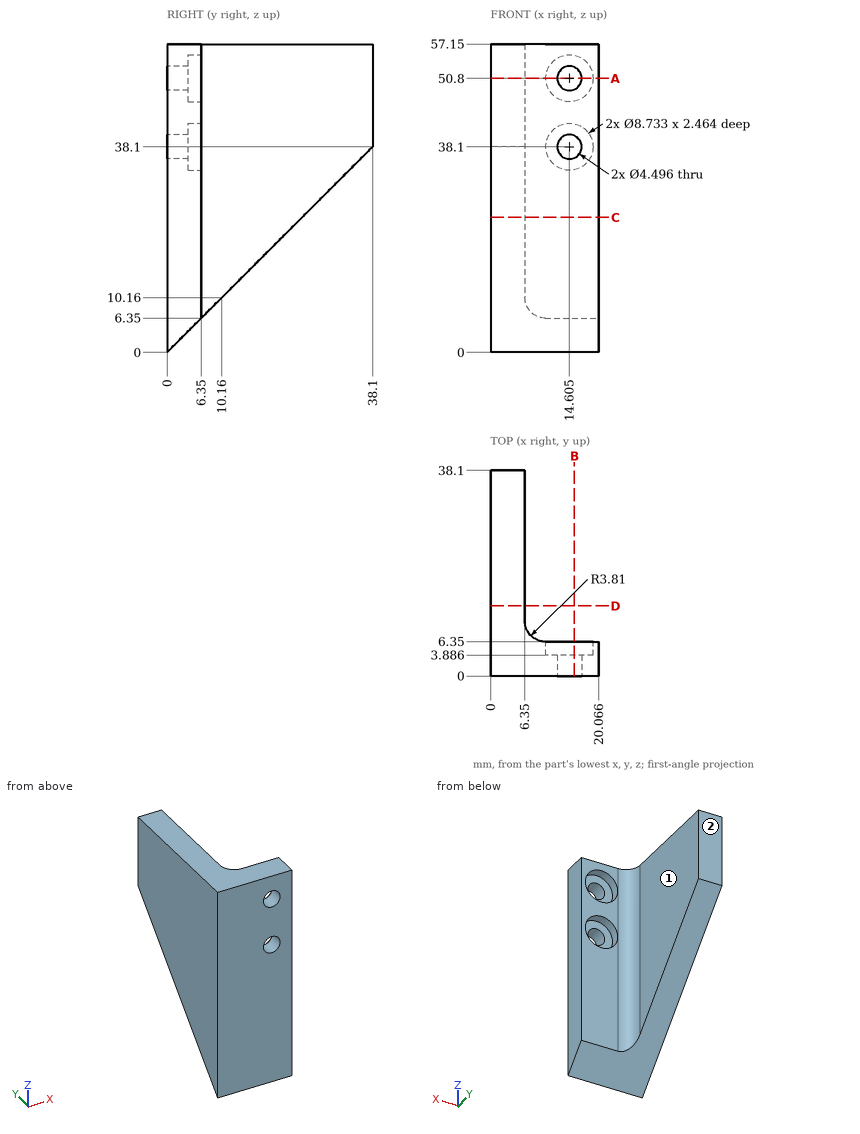
Could you check a few things on this drawing? It's one solid part, dimensions in mm from its lowest x, y, z. A direction names the side the tool comes from. Give positions to 0.01 mm unless a question says otherwise; leave off trailing zeros. Write each loop counter-clockwise with the first axis right and the second up, starting at its lowest first coordinate (ties: lowest second). Pieces come first, ordered by that corner, then holes. Notation, with made-up numbers: (76.5, 10.5) - (85.5, 10.5) arc R26 cw to (85.5, 46.5) - close; hole circle Ø10 at (33, 21). An arc over 180 degrees is marked (long way). Use CSV: the item, a comma, the result in double quotes. Start each with the question number.
Item 1: If I drill on line 1 along X through (y, z) = (5, 38); line 2 along X through (y, z) = (2.1, 38.1); line 3 along Y through (x, z) = (17.25, 32.5), over which ranges is the centre line in solid material (lowest first)?
Item 2: I want a section at D-D, the plane y = 13. Please give me the cut outline in (x, z), then the cut area to 3 significant figures.
Item 3: I want a section at A-A, the plane z = 50.8. Please give me the cut outline in (x, y), then the cut area to 3 significant figures.
Item 4: I want a section at B-B, the plane x = 15.5. Please give me the cut outline in (y, z).
Item 5: I'm going to push flat-ended pins straight in: pin 1 (14 mm diameter, centred on y = 27.5, z = 22.5, fed in from +X); pin 2 (9.5 mm diameter, centred on x = 14.5, z = 49, fed in from +Y); pin 3 (9.5 mm diameter, centred on x = 14, z = 37, fed in from +Y). Where does each tip first touch, or does it pass through?
Item 6: I want a section at C-C, the plane z = 25. Please give me the cut outline in (x, y).
Item 7: For the marked faces 1 and 2, which set-ups out of +Z, -Z, +X, -X, +Y, -Y let a thin tool reach every point of the face, with its end or its side?
Findings:
1,line 1,"x = 0 to 10.24, 18.97 to 20.07"
1,line 2,"x = 0 to 12.36, 16.85 to 20.07"
1,line 3,"y = 0 to 6.35"
2,outline,"(0, 13) - (6.35, 13) - (6.35, 57.15) - (0, 57.15) - close"
2,area,"280 mm2"
3,outline,"(0, 0) - (12.36, 0) - (12.36, 3.89) - (10.24, 3.89) - (10.24, 6.35) - (10.16, 6.35) arc R3.81 cw to (6.35, 10.16) - (6.35, 38.1) - (0, 38.1) - close; (16.85, 0) - (20.07, 0) - (20.07, 6.35) - (18.97, 6.35) - (18.97, 3.89) - (16.85, 3.89) - close"
3,area,"293 mm2"
4,outline,"(0, 0) - (6.35, 6.35) - (6.35, 33.83) - (3.89, 33.83) - (3.89, 36.04) - (0, 36.04) - close; (0, 40.16) - (3.89, 40.16) - (3.89, 42.37) - (6.35, 42.37) - (6.35, 46.53) - (3.89, 46.53) - (3.89, 48.74) - (0, 48.74) - close; (0, 52.86) - (3.89, 52.86) - (3.89, 55.07) - (6.35, 55.07) - (6.35, 57.15) - (0, 57.15) - close"
5,pin 1,"stops at x = 6.35"
5,pin 2,"stops at y = 6.37"
5,pin 3,"stops at y = 6.46"
6,outline,"(0, 0) - (20.07, 0) - (20.07, 6.35) - (10.16, 6.35) arc R3.81 cw to (6.35, 10.16) - (6.35, 25) - (0, 25) - close"
7,face 1,"+Z, -Z, +X, +Y"
7,face 2,"+Z, -Z, +X, -X, +Y"
